Can you work these out from the model? Positions are in its coordinate system, mm. Face numbers are marked on the shaded views. Coordinates: 2 decimals unless noted, no trailing zeros. Order: outer loops, then holes, each group sorted by start corner. A loop starts at its lowest first (then second) coordinate and runs counter-clockwise, first axis right, second up. Notation, with made-up numbers: (4, 18.25) -> (51, 18.25) arc R8 cw to (51, 22.25) -> close; hole circle Ø2 at (82, -12.75). An arc over 180 degrees is marked (long way). Answer as a JSON object with one key per item and string values. Group by question number.
(1) I want a section at B-B, the plane y = 0. List the corners of the cut face in (x, z) for me.
(2) I need wall thicknesses on line 1 (Z direction, x = 3, y = -0.25); line 2 (Z direction, x = 0.75, y = -0.25); line 3 (X direction, y = -3.25, z = 5.25). Which ranges of each line are inside material? Lowest first, please.
(3) If we mould it in two halves opening along X, with no side actions, what happens to the marked faces 1, 2 and 3? For each: pulls with the +X half, pulls with the -X half, needs draft (parallel to the pull), parting line crosses it, or undercut.
(4) I want a section at A-A, the plane x = 0. List the corners of the cut face in (y, z) for me.
(5) I want a section at C-C, the plane z = 1.25. List the corners of the cut face in (x, y) for me.
(6) For pin 1 (1 mm diameter, centred on x = 0, y = 0.5, fed in from -Z); pin 2 (1.5 mm diameter, centred on y = -2.5, z = 3, fed in from -X); pin 3 (2 mm diameter, centred on x = -1.5, z = 1.5, fed in from -Y), each with a flat end and sliding along its axis, tell me the tip position at first contact or that it passes through.
from build123d import *

# Parameters (mm, degrees)
CYLINDER002_R     = 0.3
CYLINDER002_DEPTH = 3.1
CYLINDER003_R     = 0.3
CYLINDER003_DEPTH = 3.1
CYLINDER001_R     = 1.6
CYLINDER001_DEPTH = 0.5
CYLINDER_R        = 4.25
CYLINDER_DEPTH    = 7.5
FILLET_R          = 0.2


with BuildPart() as pin1:
    # Cylinder002 → Cylinder002 (new body)
    with BuildSketch(Plane(origin=(-2.54, 0, -2.6), x_dir=(1, 0, 0), z_dir=(0, 0, 1))):
        Circle(CYLINDER002_R)
    extrude(amount=CYLINDER002_DEPTH)


with BuildPart() as pin2:
    # Cylinder003 → Cylinder003 (new body)
    with BuildSketch(Plane(origin=(2.54, 0, -2.6), x_dir=(1, 0, 0), z_dir=(0, 0, 1))):
        Circle(CYLINDER003_R)
    extrude(amount=CYLINDER003_DEPTH)


with BuildPart() as fuss:
    # Cylinder001 → Cylinder001 (new body)
    with BuildSketch(Plane.XY):
        Circle(CYLINDER001_R)
    extrude(amount=CYLINDER001_DEPTH)


with BuildPart() as obj1:
    # Cylinder → Cylinder (new body)
    with BuildSketch(Plane.XY.offset(0.5)):
        Circle(CYLINDER_R)
    extrude(amount=CYLINDER_DEPTH)

    # Fusion: union Fuss
    add(fuss.part)

    # Fillet
    fillet_edges = [obj1.edges().sort_by_distance(p)[0] for p in [
        (-4.25, 0, 8),
    ]]
    fillet(fillet_edges, radius=FILLET_R)

    # Fusion001: union pin1, pin2
    add(pin1.part)
    add(pin2.part)


solid = obj1.part
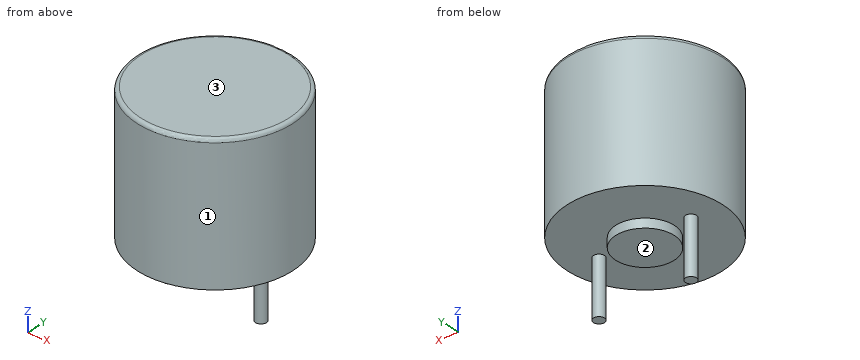
Computed values:
{
 "1": {"outline": "(-4.25, 0.5) -> (-2.84, 0.5) -> (-2.84, -2.6) -> (-2.24, -2.6) -> (-2.24, 0.5) -> (-1.6, 0.5) -> (-1.6, 0) -> (1.6, 0) -> (1.6, 0.5) -> (2.24, 0.5) -> (2.24, -2.6) -> (2.84, -2.6) -> (2.84, 0.5) -> (4.25, 0.5) -> (4.25, 7.8) arc R0.2 ccw to (4.05, 8) -> (-4.05, 8) arc R0.2 ccw to (-4.25, 7.8) -> close"},
 "2": {"line 1": "z = 0.5 to 8", "line 2": "z = 0 to 8", "line 3": "x = -2.74 to 2.74"},
 "3": {"face 1": "parting line crosses it", "face 2": "undercut", "face 3": "needs draft"},
 "4": {"outline": "(-4.25, 0.5) -> (-1.6, 0.5) -> (-1.6, 0) -> (1.6, 0) -> (1.6, 0.5) -> (4.25, 0.5) -> (4.25, 7.8) arc R0.2 ccw to (4.05, 8) -> (-4.05, 8) arc R0.2 ccw to (-4.25, 7.8) -> close"},
 "5": {"outline": "circle Ø8.5 at (0, 0)"},
 "6": {"pin 1": "stops at z = 0", "pin 2": "stops at x = -3.87", "pin 3": "stops at y = -4.22"}
}
